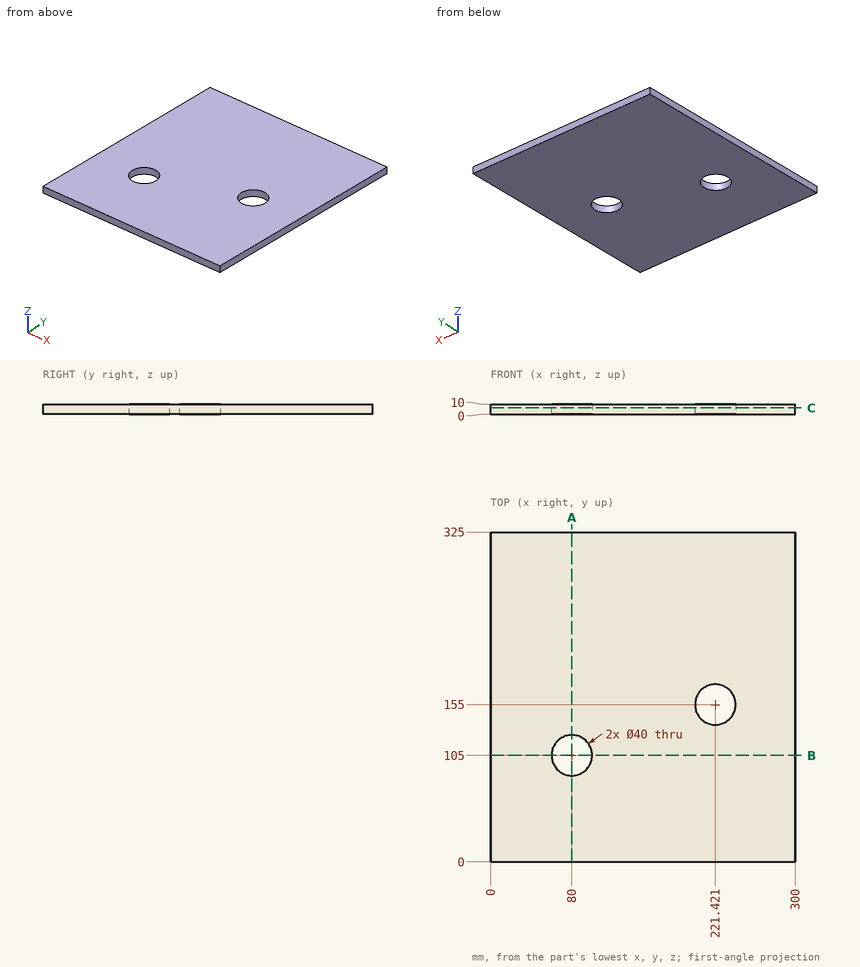
Geometry: see drawing. Coordinates: mm, zero at the bounding-box minimum. Coordinates: 2 decimals unless noted, no trailing zeros. Order: outer loops, then holes, each group sorted by start corner. A loop starts at its lowest first (then second) coordinate and runs counter-clockwise, first axis right, second up. Notation, with made-up numbers: (-22.5, 30.25) - (-10.5, 30.25) arc R10 cw to (-10.5, 49.25) - close; hole circle Ø8 at (40, 56.25). An arc over 180 degrees is marked (long way). Return JSON: item names as keys, results as strings.
Q1. Cut plane B-B (y = 105). Return loops of the section in (x, z), then the cut area to 3 significant figures.
The answers:
{"outline": "(0, 0) - (60, 0) - (60, 10) - (0, 10) - close; (100, 0) - (300, 0) - (300, 10) - (100, 10) - close", "area": "2,600 mm2"}
Q2. Cut plane C-C (z = 6.25). Return loops of the section in (x, y).
The answers:
{"outline": "(0, 0) - (300, 0) - (300, 325) - (0, 325) - close; hole circle Ø40 at (80, 105); hole circle Ø40 at (221.42, 155)"}
Q3. Cut plane A-A (x = 80). Return loops of the section in (y, z), then the cut area to 3 significant figures.
The answers:
{"outline": "(0, 0) - (85, 0) - (85, 10) - (0, 10) - close; (125, 0) - (325, 0) - (325, 10) - (125, 10) - close", "area": "2,850 mm2"}
Q4. Ray query, probe 1 along Y at (x, z) = (80, 6.5); probe 2 along X at (y, z) = (110, 9) (1 decimal); probe 3 along X at (y, z) = (111, 5.5). Return the intervals inside material, ascending.
The answers:
{"probe 1": "y = 0 to 85, 125 to 325", "probe 2": "x = 0 to 60.6, 99.4 to 300", "probe 3": "x = 0 to 60.92, 99.08 to 300"}
